```python
from build123d import *

# Parameters (mm, degrees)
F1_DEPTH      = 44
F2_R          = 5.5
F3_DEPTH      = 44.001
F4_W          = 33
F4_H          = 19
F5_DEPTH      = 24.001
F5_DEPTH_BACK = 25
F8_DEPTH      = 24


with BuildPart() as f1:
    # F0 (on Front) → F1 (new body)
    with BuildSketch(Plane.XZ):
        with BuildLine():
            Line((-29, -34), (0, 0))
            Line((0, 0), (0, 19))
            Line((0, 19), (-5, 24))
            Line((-5, 24), (-34, 24))
            ThreePointArc((-34, 24), (-42.4407650408, 15.0219737764), (-54.6144594201, 13.1107871023))
            Line((-54.6144594201, 13.1107871023), (-71, 16))
            Line((-71, 16), (-78, 16))
            Line((-78, 16), (-85, 9))
            Line((-85, 9), (-85, 0))
            Line((-85, 0), (-85, -9))
            Line((-85, -9), (-78, -16))
            Line((-78, -16), (-73.6665455603, -16.8407740419))
            Line((-73.6665455603, -16.8407740419), (-42.1131182037, -16.8407740419))
            ThreePointArc((-42.1131182037, -16.8407740419), (-38.6217617691, -18.2616079035), (-37.1146603126, -21.7166019433))
            ThreePointArc((-37.1146603126, -21.7166019433), (-35.7621956578, -28.2996251104), (-32.2025494985, -34))
            Line((-32.2025494985, -34), (-29, -34))
        make_face()
        with BuildLine():
            ThreePointArc((-64, -3.0970651257), (-66.5465131336, -8.4976627528), (-72.3332727801, -9.9689195838))
            ThreePointArc((-72.3332727801, -9.9689195838), (-75.4534868664, 2.3035325015), (-64, -3.0970651257))
        make_face(mode=Mode.SUBTRACT)
    extrude(amount=F1_DEPTH)

    # F2 (on face) → F3 (cut, through all)
    with BuildSketch(Plane.XZ.offset(44)):
        with Locations((-15.9680212459, 10)):
            Circle(F2_R)
    extrude(amount=-F3_DEPTH, mode=Mode.SUBTRACT)

    # F4 (on Top) → F5 (cut, two sides)
    with BuildSketch(Plane.XY) as f5_sk:
        with Locations((-68.5, -34.5)):
            Rectangle(F4_W, F4_H)
    extrude(amount=F5_DEPTH, mode=Mode.SUBTRACT)
    extrude(f5_sk.sketch, amount=-F5_DEPTH_BACK, mode=Mode.SUBTRACT)

    # F7 (on offset) → F8 (cut)
    with BuildSketch(Plane(origin=(0, -12, 0), x_dir=(-1, 0, 0), z_dir=(0, 1, 0))):
        with BuildLine():
            Line((0, 0), (10.2352941176, -12))
            ThreePointArc((10.2352941176, -12), (28.7839327574, -1.495476016), (39.5518853442, 16.901486141))
            ThreePointArc((39.5518853442, 16.901486141), (36.348995532, 20.1168194328), (34, 24))
            Line((34, 24), (5, 24))
            Line((5, 24), (0, 19))
            Line((0, 19), (0, 0))
        make_face()
    extrude(amount=-F8_DEPTH, mode=Mode.SUBTRACT)


solid = f1.part
```
CAD build for the part. Positions are in the model's coordinates, mm. A direction names the side the tool comes from. Give positions to 0.01 mm unless a question says otherwise; leave off trailing zeros. Loops run counter-clockwise (first coordinate to the right, second up) from the corner with the lowest first, then second, coordinate; pieces in that order, holes last. Notation, with made-up numbers: (80.25, -13.5) -> (109.25, -13.5) arc R19 cw to (109.25, -0.5) -> close; hole circle Ø11 at (-36.75, 71). An arc over 180 degrees is marked (long way). Use a Markdown table: item, result.
1. Slice it at B-B (z = 1). List the corners of the cut face in (x, y), plus the area to 3 significant figures.
Check result:
| item | result |
|---|---|
| outline | (-85, -25) -> (-76.68, -25) -> (-76.68, 0) -> (-85, 0) -> close; (-65.32, -25) -> (-52, -25) -> (-52, -44) -> (0, -44) -> (0, -36) -> (-31.11, -36) -> (-31.11, -12) -> (0, -12) -> (0, 0) -> (-65.32, 0) -> close |
| area | 2,080 mm^2 |
2. Mould opens along X. For faces 4 (the flat face through (-75.864, -12.325, -16.415)), 5 (the flat face through (-19, -6, 24)), 6 (the cylindrical face through (-10.89, -6.08, 7.89)) say: pulls with the +X half, pulls with the -X half, needs draft (parallel to the pull), parting line crosses it, or undercut.
Check result:
| item | result |
|---|---|
| face 4 | pulls with the -X half |
| face 5 | needs draft |
| face 6 | undercut |
3. Flat gauge pins, fed straight in: pin 1 (10 mm diameter, centred on x = -71.5, z = 8, fed in from -Y); pin 2 (5 mm diameter, centred on x = -23, y = -17, fed in from +Z); pin 3 (16 mm diameter, centred on x = -52, y = -17, fed in from -Z). Where does each tip first touch, or does it go through?
Check result:
| item | result |
|---|---|
| pin 1 | stops at y = -25 |
| pin 2 | stops at z = -4.4 |
| pin 3 | stops at z = -16.84 |
4. Slice it at A-A (y = -9.5). List the corners of the cut face in (x, z), plus the area to 3 significant figures.
Check result:
| item | result |
|---|---|
| outline | (-85, -9) -> (-78, -16) -> (-73.67, -16.84) -> (-42.11, -16.84) arc R5 cw to (-37.11, -21.72) arc R19 ccw to (-32.2, -34) -> (-29, -34) -> (0, 0) -> (0, 19) -> (-5, 24) -> (-34, 24) arc R19 cw to (-54.61, 13.11) -> (-71, 16) -> (-78, 16) -> (-85, 9) -> close; hole circle Ø14 at (-71, -3.1); hole circle Ø11 at (-15.97, 10) |
| area | 2,840 mm^2 |
5. Which spindle directions (+Z, -Z, +X, -X, +Y, -Y) get a long thin tool onto all of the face, cutting with end or side? Do faces 1 (the flat face through (-65, -25, 3)), 2 (the flat face through (-62.693, -12.325, 14.535)), 3 (the flat face through (-55, -17, -16.841)). Say none if no direction does.
Check result:
| item | result |
|---|---|
| face 1 | +Z, -Z, -X, -Y |
| face 2 | +Z, +Y, -Y |
| face 3 | -Z, -X, +Y, -Y |
6. Slice it at C-C (x = -77). List the corners of the cut face in (y, z).
Check result:
| item | result |
|---|---|
| outline | (-25, -16.19) -> (0, -16.19) -> (0, -6.7) -> (-25, -6.7) -> close; (-25, 0.51) -> (0, 0.51) -> (0, 16) -> (-25, 16) -> close |
7. Wall check: L1, parallel to Y at x = -13, z = 17.5; L2, parallel to Z at x = -71, y = -10; L3, parallel to Y at x = -73, z = -10.5. Give the ranges that are in metal, low to high. Write a range as [from, to].
Check result:
| item | result |
|---|---|
| L1 | y = [-44, -36], [-12, 0] |
| L2 | z = [-16.84, -10.1], [3.9, 16] |
| L3 | y = [-25, 0] |
8. Slice it at D-D (y = -26). List the corners of the cut face in (x, z).
Check result:
| item | result |
|---|---|
| outline | (-52, -16.84) -> (-42.11, -16.84) arc R5 cw to (-37.11, -21.72) arc R19 ccw to (-32.2, -34) -> (-29, -34) -> (-10.24, -12) arc R41 cw to (-39.55, 16.9) arc R19 cw to (-52, 12.83) -> close |
